Geometry check sheet. Reference: drawing and pictorial views, mm from the part's lowest x, y, z. Round coordinates to 2 decimals unless told otherwise and drop trailing zeros. Loops run counter-clockwise (first coordinate to the right, second up) from the corner with the lowest first, then second, coordinate; pieces in that order, holes last. Notation, with made-up numbers: (36, -0.75) - (90, -0.75) arc R21 ccw to (90, 37.25) - close; hole circle Ø1 at (15.25, 43.25). An arc over 180 degrees is marked (long way). Put each result on its own line as item: value. Start each with the question number.
Item 1: Section check A-A, the plane x = 72.5. Record the cut outline in (y, z).
Item 2: Material ranges on line 1 along Z through (x, y) = (75, 83), recorded low to high.
Item 3: Draft check along X on the marked faces 1, 2, 3 and 4. Enter one of: pulls with the +X half, pulls with the -X half, needs draft (parallel to the pull), parting line crosses it, or undercut.
Item 4: Gauge pin test, flat ends, axial feed: pin 1 Ø8 at (x, y) = (22.5, 59.5) entering from -Z; pin 2 Ø12 at (x, y) = (26.5, 31.5) entering from +Z. Record the tip position at first contact, or that the pin passes through.
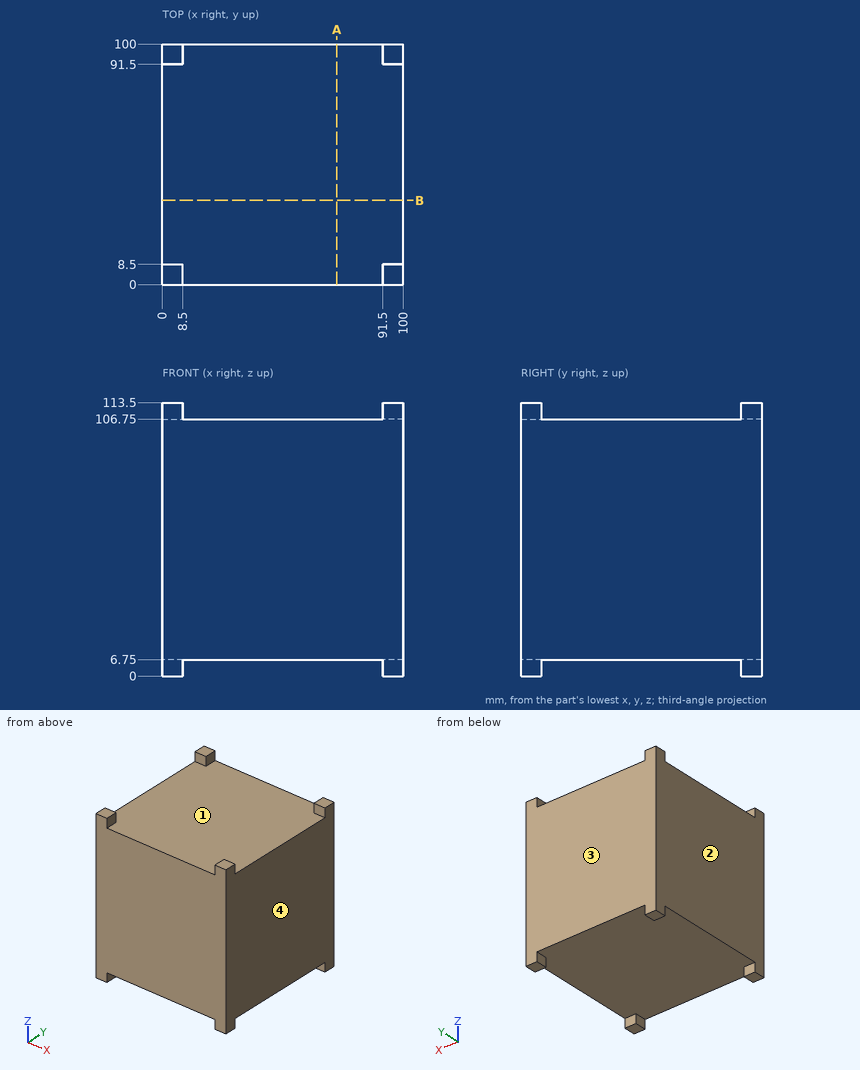
Check result:
1. outline: (0, 6.75) - (100, 6.75) - (100, 106.75) - (0, 106.75) - close
2. line 1: 6.75 to 106.75
3. face 1: undercut
3. face 2: pulls with the -X half
3. face 3: needs draft
3. face 4: pulls with the +X half
4. pin 1: z = 6.75
4. pin 2: z = 106.75
